Source: CAD feature listing. Evaluate the final solid. Frame: model axes, mm. A direction names the side the tool comes from. Coordinates: 2 decimals unless noted, no trailing zeros. Write each loop counter-clockwise with the first axis right and the second up, starting at its lowest first coordinate (ties: lowest second). Pieces come first, ordered by that corner, then holes. Notation, with made-up numbers: M 67.25,-20.5 L 121.25,-20.5 A22 cw 121.25,3.5 Z; hole C 68.5,-2 d2. An arc over 180 degrees is marked long. Write item = value, one per line. Start each with the question number.
1. Section query A-A (y = 0.4). Give the number of separate pieces and of enclosed holes in the cut face, then the cut area to 3 significant figures.
2. Section query C-C (x = 41). Output: boundary loops of the cut face in (y, z).
3. Line query: line 1 along X through (y, z) = (0, 1.3); line 2 along X through (y, z) = (-0.5, 0.7); line 3 along X through (y, z) = (-2.4, 1.6). Output: solid intervals per line, ascending.
4. Section query B-B (x = 21). Output: boundary loops of the cut face in (y, z), then the cut area to 3 significant figures.
5. Pull-direction query (Y, two-part tool) for faces 4 (the face through (10.8, -0.54, -2.44)), 5 (the face through (8.768, 0.27, 2.183)), 6 (the face through (0, 0, 0)), 7 (the face through (40.325, 0.43, 0.032)); classes: pulls with the +Y half, pulls with the -Y half, needs draft (parallel to the pull), parting line crosses it, or undercut.
6. Pin query (flat end, axial travel): pin 1 Ø2 at (x, y) = (18, 1) entering from -Z; pin 2 Ø3.5 at (x, y) = (1.5, 0) entering from -Z; pin 3 Ø0.7 at (y, z) = (2, -1.5) entering from -X. Return the tip coordinate at first contact, or that it passes through.
7. Access query for faces 1 (the face through (2, 0, -0.75)), 2 (the face through (30.964, 2.146, 0.676)), 3 (the face through (8.768, -2.026, -0.857)). Directions: +Z, -Z, +X, -X, +Y, -Y. A direction counts if a zero-diameter tool reaches every point of the face in a straight line with its end or side. Return the directions, or none.
Autodesk Inventor part; units mm, degrees
ref_plane "Work Plane1" through (30.75, 0, -2.25) normal (0, 0, 1) x (1, 0, 0)
ref_plane "YZ Plane" through (0, 0, 0) normal (1, 0, 0) x (0, 1, 0)
ref_plane "XZ Plane" through (0, 0, 0) normal (0, 1, 0) x (-1, 0, 0)
sketch "Sketch1" plane through (0, 0, 0) normal (0, 0, 1) x (1, 0, 0)
  line L0 (7.5, 2.5) -> (14, 2.5)
  line L1 (15.5, 2.25) -> (46, 2.25)
  line L2 (46, 2.25) -> (46, 2)
  line L3 (46, 2) -> (48.5, 2)
  line L4 (7.5, 2.5) -> (7.5, 2)
  line L5 (7.5, 2) -> (5, 2)
  line L6 (0, 0) -> (48.5, 0)
  line L7 (48.5, 0) -> (48.5, 2)
  line L8 (14, 2.5) -> (14, 2.95)
  line L9 (14, 2.95) -> (15.5, 2.95)
  line L10 (15.5, 2.95) -> (15.5, 2.25)
  line L11 (5, 2) -> (5, 1.75)
  line L12 (5, 1.75) -> (0, 1.75)
  line L13 (0, 1.75) -> (0, 0)
  dimension "d37" = 3.7
  dimension "d45" = 7.34
  dimension "d4" = 2.5
  dimension "d5" = 4.5
  dimension "d6" = 5
  dimension "d7" = 4
  dimension "d8" = 4
  dimension "d12" = 32
  dimension "d13" = 6.5
  dimension "d14" = 1.5
  dimension "d15" = 5.9
  dimension "d25" = 2.5
  dimension "d26" = 5
  dimension "d27" = 3.5
revolve "Revolution1" add sketch "Sketch1" angle 360 about axis through (0, 0, 0) along (1, 0, 0)
ref_plane "Work Plane1" through (30.75, 0, -2.25) normal (0, 0, 1) x (1, 0, 0)
sketch "Sketch2" plane through (30.75, 0, -2.25) normal (0, 0, 1) x (1, 0, 0)
  line L0 (-16.75, -2.95) -> (-16.75, 2.95)
  line L1 (-30.75, 0) -> (16.721, 0) construction
  point P0 (1.25, 0)
  point P1 (10.25, 0)
  dimension "d16" = 18
  dimension "d17" = 27
hole "Hole1" at (32, 0, -2.25) at (41, 0, -2.25) direction (0, 0, 1) diameter 1.6 end through all
sketch "Sketch4" plane through (14, 0, 0) normal (-1, 0, 0) x (0, 0, 1)
  line L0 (0.75, -2.95) -> (-0.75, -2.95)
  line L1 (-0.75, -2.95) -> (-0.75, -10)
  line L2 (-0.75, -10) -> (0.75, -10)
  line L3 (0.75, -10) -> (0.75, -2.95)
  line L4 (0, 0) -> (0, -9.1569) construction
  dimension "d28" = 1.5
  dimension "d29" = 2.95
  dimension "d30" = 10
extrude "Extrusion1" [suppressed]
pattern_circular "Circular Pattern1" [suppressed]
sketch "Sketch5" plane through (7.5, 0, 0) normal (-1, 0, 0) x (0, 0, 1)
  line L0 (1.4255, 3.4144) -> (3.6697, 0.4727) construction
  line L1 (3.6697, 0.4727) -> (2.2442, -2.9417) construction
  line L2 (2.2442, -2.9417) -> (-1.4255, -3.4144) construction
  line L3 (-1.4255, -3.4144) -> (-3.6697, -0.4727) construction
  line L4 (-3.6697, -0.4727) -> (-2.2442, 2.9417) construction
  line L5 (-2.2442, 2.9417) -> (1.4255, 3.4144) construction
  line L6 (0, 0) -> (11.1686, 0) construction
  dimension "d37" = 3.7
  dimension "d45" = 7.34
hole "Hole2" at (7.5, -3.4144, -1.4255) at (7.5, 0.4727, 3.6697) at (7.5, 2.9417, -2.2442) direction (1, 0, 0) diameter 3 depth 2.5
sketch "Sketch6" plane through (0, 0, 0) normal (-1, 0, 0) x (0, 0, 1)
  circle A0 centre (0, 0) radius 1.75
  line L0 (-0.75, -1.5811) -> (-0.75, 1.5811)
  dimension "d46" = 0.75
extrude "Extrusion2" cut sketch "Sketch6" against normal up to surface (5 mm away) contours L0 A0 picked at (-1.0833, 0)
properties part number "thumb_03 CMC shaft" material "Stainless Steel"
Results are:
q1.separate_pieces = 3
q1.enclosed_holes = 0
q1.area = 195 mm^2
q2.outline = M -0.8,-2.1 L -0.8,2.1 A2.25 ccw Z; M 0.8,-2.1 A2.25 ccw 0.8,2.1 Z
q3.line_1 = 0 to 31.2, 32.8 to 40.2, 41.8 to 48.5
q3.line_2 = 0 to 31.38, 32.62 to 40.38, 41.62 to 48.5
q3.line_3 = 14 to 15.5
q4.outline = C 0,0 d4.5
q4.area = 15.9 mm^2
q5.face_4 = parting line crosses it
q5.face_5 = undercut
q5.face_6 = needs draft
q5.face_7 = undercut
q6.pin_1 = -2.25
q6.pin_2 = -0.75
q6.pin_3 = 7.5
q7.face_1 = -Z, -X, +Y, -Y
q7.face_2 = +X
q7.face_3 = -X, -Y
